from build123d import *

# Parameters (mm, degrees)
SKETCH1_W           = 17
SKETCH1_H           = 21.5
BOSS_EXTRUDE1_DEPTH = 11.5
SKETCH2_R           = 3.5
BOSS_EXTRUDE2_DEPTH = 16
SKETCH3_R           = 3.5
BOSS_EXTRUDE3_DEPTH = 6
CHAMFER1_SIZE       = 3


with BuildPart() as part:
    # Sketch1 → Boss-Extrude1 (new body)
    with BuildSketch(Plane(origin=(0, 0, 0), x_dir=(1, 0, 0), z_dir=(0, 1, 0))):
        with Locations((8.5, 10.75)):
            Rectangle(SKETCH1_W, SKETCH1_H)
    extrude(amount=BOSS_EXTRUDE1_DEPTH)

    # Sketch2 → Boss-Extrude2 (add)
    with BuildSketch(Plane(origin=(0, 11.5, 0), x_dir=(1, 0, 0), z_dir=(0, 1, 0))):
        with Locations(Location((8.5, 15.5, 0), (0, 0, 90))):
            Circle(SKETCH2_R)
    extrude(amount=BOSS_EXTRUDE2_DEPTH)

    # Sketch3 → Boss-Extrude3 (add)
    with BuildSketch(Plane.XZ):
        with Locations(Location((8.5, -6, 0), (0, 0, 270))):
            Circle(SKETCH3_R)
    extrude(amount=BOSS_EXTRUDE3_DEPTH)

    # Chamfer1
    chamfer1_edges = [part.edges().sort_by_distance(p)[0] for p in [
        (8.5, -6, -2.5),
    ]]
    chamfer(chamfer1_edges, length=CHAMFER1_SIZE)


solid = part.part
For this review, take the finished solid that the model builds, in its own axes (mm). A direction names the side the tool comes from. Round coordinates to 2 decimals unless told otherwise and drop trailing zeros. Order: outer loops, then holes, each group sorted by start corner. A loop starts at its lowest first (then second) coordinate and runs counter-clockwise, first axis right, second up. Notation, with made-up numbers: M 68.25,21 L 112.25,21 A28 cw 112.25,39 Z; hole C 11,53.25 d2. An arc over 180 degrees is marked long. Use a Markdown table: item, result. Add a question column.
Item 1: To check wall thickness, follow line 1 along X through (y, z) = (20.5, -15.25); line 2 along Y through (x, z) = (4.5, -4); line 3 along Y through (x, z) = (10.75, -14.75). State the ranges of each line that lie inside material, in increasing order.
Item 2: Add section D-D, the plane z = -6. Give the boundary of the cut face in (x, y).
Item 3: Add section A-A, the plane z = -15.5. Give the boundary of the cut face in (x, y), then the cut area to 4 significant figures.
Item 4: Tool access review of faces 1 (the cylindrical face through (5.395, -1.479, -7.615)), 2 (the cylindrical face through (9.841, 19.388, -18.733)), 3 (the flat face through (0, 6, -11)): name each direction out of +Z, -Z, +X, -X, +Y, -Y from which nothing blocks a thin tool from reaching the whole face with its end or side.
Item 5: Add section B-B, the plane x = 8.5. Give the boundary of the cut face in (y, z), then the cut area to 3 significant figures.
Item 6: Insertion check: pin 1 (1 mm diameter, centred on x = 10, y = -2.5, fed in from -Z); pin 2 (8 mm diameter, centred on y = 14, z = -15.5, fed in from +X); pin 3 (5 mm diameter, centred on x = 7.5, y = 21, fed in from -Z); pin 4 (5 mm diameter, centred on x = 5, z = -3, fed in from -Y). Each pin has a flat end and moves straight along its axis. Give the tip position at first contact, or say it passes through.
Item 7: Add section C-C, the plane y = 14. Give the boundary of the cut face in (x, z), then the cut area to 3 significant figures.
Geometry results:
| question | item | result |
|---|---|---|
| 1 | line 1 | x = 5.01 to 11.99 |
| 1 | line 2 | y = 0 to 11.5 |
| 1 | line 3 | y = 0 to 27.5 |
| 2 | outline | M 0,0 L 5,0 L 5,-3 L 8,-6 L 9,-6 L 12,-3 L 12,0 L 17,0 L 17,11.5 L 0,11.5 Z |
| 3 | outline | M 0,0 L 17,0 L 17,11.5 L 12,11.5 L 12,27.5 L 5,27.5 L 5,11.5 L 0,11.5 Z |
| 3 | area | 307.5 mm² |
| 4 | face 1 | -Y |
| 4 | face 2 | +Y |
| 4 | face 3 | +Z, -Z, -X, +Y, -Y |
| 5 | outline | M -6,-6.5 L -3,-9.5 L 0,-9.5 L 0,-21.5 L 11.5,-21.5 L 11.5,-19 L 27.5,-19 L 27.5,-12 L 11.5,-12 L 11.5,0 L 0,0 L 0,-2.5 L -3,-2.5 L -6,-5.5 Z |
| 5 | area | 392 mm² |
| 6 | pin 1 | stops at z = -9.35 |
| 6 | pin 2 | stops at x = 17 |
| 6 | pin 3 | stops at z = -19 |
| 6 | pin 4 | stops at y = -4.39 |
| 7 | outline | C 8.5,-15.5 d7 |
| 7 | area | 38.5 mm² |
